```python
from build123d import *

# Parameters (mm, degrees)
F0_R     = 10
F1_DEPTH = 30


with BuildPart() as f1:
    # F0 (on Front) → F1 (new body)
    with BuildSketch(Plane.XZ):
        Polygon((-43.386797, 55.138951), (-53.386797, 45.138951), (-93.386797, 45.138951), (-93.386797, -54.861049), (-53.386797, -54.861049), (-43.386797, -64.861049), (-43.386797, -70.548529), (66.613203, -70.548529), (76.613203, -70.548529), (76.613203, -64.861049), (76.613203, -60.548529), (76.613203, -54.861049), (86.613203, -54.861049), (96.613203, -54.861049), (106.613203, -54.861049), (106.613203, -44.861049), (106.613203, 35.138951), (106.613203, 45.138951), (96.613203, 45.138951), (86.613203, 45.138951), (76.613203, 55.138951), (76.613203, 59.451471), (76.613203, 69.451471), (66.613203, 69.451471), (-33.386797, 69.451471), (-43.386797, 69.451471), (-43.386797, 59.451471), align=None)
        Polygon((-81.881762, -44.861049), (-81.881762, -24.861049), (-51.881762, -24.861049), (-41.881762, -24.861049), (-41.881762, -34.861049), (-51.881762, -44.861049), align=None, mode=Mode.SUBTRACT)
        Polygon((-81.881762, -14.861049), (-81.881762, 5.138951), (-51.881762, 5.138951), (-41.881762, 5.138951), (-41.881762, -4.861049), (-41.881762, -14.861049), align=None, mode=Mode.SUBTRACT)
        with Locations((86.613203, -34.861049)):
            Circle(F0_R, mode=Mode.SUBTRACT)
        with Locations((86.613203, -4.861049)):
            Circle(F0_R, mode=Mode.SUBTRACT)
        Polygon((-81.881762, 15.138951), (-81.881762, 35.138951), (-51.881762, 35.138951), (-41.881762, 25.138951), (-41.881762, 15.138951), align=None, mode=Mode.SUBTRACT)
        Polygon((-23.386797, 39.451471), (-13.386797, 49.451471), (46.613203, 49.451471), (56.613203, 39.451471), (56.613203, 24.451471), (56.613203, -0.548529), (56.613203, -40.548529), (46.613203, -50.548529), (-13.386797, -50.548529), (-23.386797, -40.548529), (-23.386797, -0.548529), (-23.386797, 24.451471), align=None, mode=Mode.SUBTRACT)
        with Locations((86.613203, 25.138951)):
            Circle(F0_R, mode=Mode.SUBTRACT)
    extrude(amount=F1_DEPTH)


solid = f1.part
```
Geometry: final body of the model. Coordinates: model frame, mm. A direction names the side the tool comes from. Round coordinates to 2 decimals unless told otherwise and drop trailing zeros. Write each loop counter-clockwise with the first axis right and the second up, starting at its lowest first coordinate (ties: lowest second). Pieces come first, ordered by that corner, then holes.
Item 1: Section query B-B (x = 27). Return loops of the section in (y, z).
Item 2: Section query C-C (z = 21). Return loops of the section in (x, y), plus the area to 3 significant figures.
Item 3: Mould query, pull axis Z, two halves, no side actions, for faces 4 (the face through (91, -15, -54.861)), 5 (the face through (-48.317, -14.79, 50.209)), 6 (the face through (-39, 0, 0)), 7 (the face through (-41.882, -15, -5)). Classes: +Z half, -Z half, draft (parallel to the pull), parting line (faces both ways), or undercut.
Item 4: Set-up query: faces 1 (the face through (76.613, -15, -63)), 2 (the face through (97, -15, 45.139)), 3 (the face through (-81.882, -15, -35)). Return all of +Z, -Z, +X, -X, +Y, -Y with unobstructed straight access to the full face (end or side cutting, diameter ignored); none if empty.
Item 5: Pin query (flat end, axial travel): P1, Ø12, axis at x = -44, z = 29, coming from the +Y side; P2, Ø12, axis at x = 86.61, z = 25.14, coming from the +Y side; P3, Ø12, axis at x = -64.5, y = -11, coming from the -Z side; P4, Ø12, axis at y = -6.5, z = 51.5, coming from the -X side. Return the tip coordinate at first contact, or that it passes through.
Item 6: Section query A-A (x = -69.5). Return loops of the section in (y, z), plus the area to 3 significant figures.
Item 7: Section query D-D (y = -20). Give the number of separate pieces and of enclosed holes in the cut face, plus the area to 3 significant figures.
Item 8: Material intervals for L1, parallel to X at y = -16.5, z = -5.5; L2, parallel to Z at x = 87.5, y = -11.5; L3, parallel to Z at x = -59.5, y = -12.5, sorted ascending.
Completed:
1. outline: (-30, -70.55) - (0, -70.55) - (0, -50.55) - (-30, -50.55) - close; (-30, 49.45) - (0, 49.45) - (0, 69.45) - (-30, 69.45) - close
2. outline: (-93.39, -30) - (-81.88, -30) - (-81.88, 0) - (-93.39, 0) - close; (-41.88, -30) - (-23.39, -30) - (-23.39, 0) - (-41.88, 0) - close; (56.61, -30) - (77.51, -30) - (77.51, 0) - (56.61, 0) - close; (95.72, -30) - (106.61, -30) - (106.61, 0) - (95.72, 0) - close
2. area: 1,850 mm2
3. face 4: -Z half
3. face 5: +Z half
3. face 6: draft
3. face 7: undercut
4. face 1: -Z, +X, +Y, -Y
4. face 2: +Z, +X, +Y, -Y
4. face 3: +Y, -Y
5. P1: stops at y = 0
5. P2: passes through
5. P3: stops at z = -54.86
5. P4: stops at x = -53.03
6. outline: (-30, -54.86) - (0, -54.86) - (0, -44.86) - (-30, -44.86) - close; (-30, -24.86) - (0, -24.86) - (0, -14.86) - (-30, -14.86) - close; (-30, 5.14) - (0, 5.14) - (0, 15.14) - (-30, 15.14) - close; (-30, 35.14) - (0, 35.14) - (0, 45.14) - (-30, 45.14) - close
6. area: 1,200 mm2
7. separate pieces: 1
7. enclosed holes: 7
7. area: 13,900 mm2
8. L1: x = -93.39 to -81.88, -41.88 to -23.39, 56.61 to 76.63, 96.59 to 106.61
8. L2: z = -54.86 to -44.82, -24.9 to -14.82, 5.1 to 15.18, 35.1 to 45.14
8. L3: z = -54.86 to -44.86, -24.86 to -14.86, 5.14 to 15.14, 35.14 to 45.14
